from build123d import *

# Parameters (mm, degrees)
F0_R           = 20
F1_DEPTH       = 39
F2_R           = 10
F3_DEPTH       = 5
F5_D           = 2.5
F5_DEPTH       = 7
F5_CSINK_D     = 4.191
F5_CSINK_ANGLE = 90
F5_TIP         = 0.7510757738


with BuildPart() as f1:
    # F0 (on Top) → F1 (new body)
    with BuildSketch(Plane.XY):
        Circle(F0_R)
    extrude(amount=F1_DEPTH)

    # F2 (on face) → F3 (join)
    with BuildSketch(Plane.XY.offset(39)):
        Circle(F2_R)
    extrude(amount=F3_DEPTH)

    # F5
    with Locations(Plane.XY.offset(39)):
        with Locations((-12.9903810568, -7.5), (12.9903810568, -7.5), (0, 15)):
            CounterSinkHole(F5_D / 2, F5_CSINK_D / 2, depth=F5_DEPTH, counter_sink_angle=F5_CSINK_ANGLE)
            with Locations((0, 0, -(F5_DEPTH + F5_TIP / 2))):  # 118° drill point
                Cone(0, F5_D / 2, F5_TIP, mode=Mode.SUBTRACT)


solid = f1.part
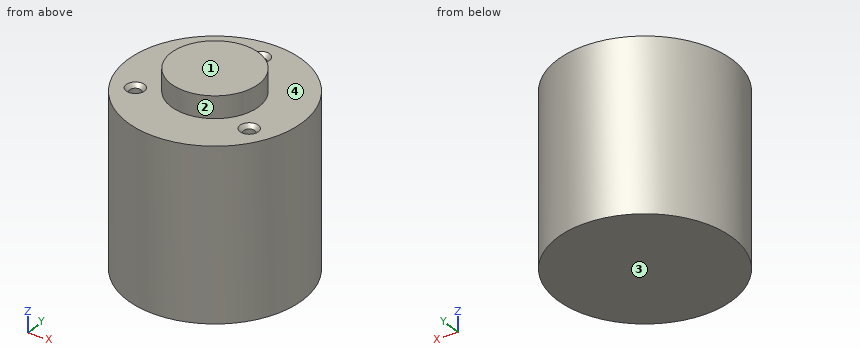
Part model, mm, in its own coordinate system. Face numbers are marked on the shaded views. A direction names the side the tool comes from. Coordinates: 2 decimals unless noted, no trailing zeros. Loops run counter-clockwise (first coordinate to the right, second up) from the corner with the lowest first, then second, coordinate; pieces in that order, holes last. Notation, with made-up numbers: (-34.75, -10.5) -> (-6.75, -10.5) arc R15 ccw to (-6.75, 15.5) -> close; hole circle Ø11 at (-9.75, 80.25). An arc over 180 degrees is marked (long way). Use a Markdown table: item, result. Add a question column.
Item 1: Probe probe 1 along Y at (x, z) = (0, 37); probe 2 along Z at (x, y) = (16, 8); probe 3 along X at (y, z) = (0.5, 35). List the from-to ranges inside material, lowest first.
Item 2: Band-saw the part on A-A on y = 0. Write the cut outline in (x, z).
Item 3: Band-saw the part on B-B on z = 25.5. Write the cut outline in (x, y).
Item 4: Band-saw the part on C-C on x = 6.5. Write the cut outline in (y, z).
Item 5: Band-saw the part on D-D on y = -12.5. Write the cut outline in (x, z), plus the area to 3 significant figures.
Item 6: Pull direction X, two halves, no side cores. Call the marked faces 1 and 2: +X half, -X half, draft (parallel to the pull), parting line (faces both ways), or undercut.
Item 7: Which spindle directions (+Z, -Z, +X, -X, +Y, -Y) get a long thin tool onto all of the face, cutting with end or side? Do the marked faces 3 and 4. Say none if no direction does.
Item 8: Flat gauge pins, fed straight in: P1, Ø2, axis at x = 5.5, y = 0, coming from the -Z side; P2, Ø8, axis at x = 16, z = 11.5, coming from the +Y side; P3, Ø3, axis at y = -6.5, z = 10, coming from the -X side; P4, Ø2, axis at x = 12.99, y = -7.5, coming from the +Z side. Where does each tip first touch, or does it go through?
Geometry says:
| question | item | result |
|---|---|---|
| 1 | probe 1 | -20 to 13.75, 16.25 to 20 |
| 1 | probe 2 | 0 to 39 |
| 1 | probe 3 | -19.99 to 19.99 |
| 2 | outline | (-20, 0) -> (20, 0) -> (20, 39) -> (10, 39) -> (10, 44) -> (-10, 44) -> (-10, 39) -> (-20, 39) -> close |
| 3 | outline | circle Ø40 at (0, 0) |
| 4 | outline | (-18.91, 0) -> (18.91, 0) -> (18.91, 39) -> (7.6, 39) -> (7.6, 44) -> (-7.6, 44) -> (-7.6, 39) -> (-18.91, 39) -> close |
| 5 | outline | (-15.61, 0) -> (15.61, 0) -> (15.61, 39) -> (-15.61, 39) -> close |
| 5 | area | 1,220 mm² |
| 6 | face 1 | draft |
| 6 | face 2 | parting line |
| 7 | face 3 | -Z, +X, -X, +Y, -Y |
| 7 | face 4 | +Z |
| 8 | P1 | z = 0 |
| 8 | P2 | y = 16 |
| 8 | P3 | x = -19.36 |
| 8 | P4 | z = 31.85 |
